The listing builds one solid part. Answer for the finished solid, in the listing's coordinates (mm). Face numbers are marked on the shaded views. A direction names the side the tool comes from. Give positions to 0.01 mm unless a question says otherwise; leave off trailing zeros. Write each loop counter-clockwise with the first axis right and the second up, starting at its lowest first coordinate (ties: lowest second). Pieces come first, ordered by that corner, then holes. Notation, with made-up numbers: (35.5, 82.5) - (70.5, 82.5) arc R20 ccw to (70.5, 103.5) - close; hole circle Ø5 at (-39, 43.5). An arc over 180 degrees is marked (long way). Answer in a Markdown table with one row per item. Add a question column.
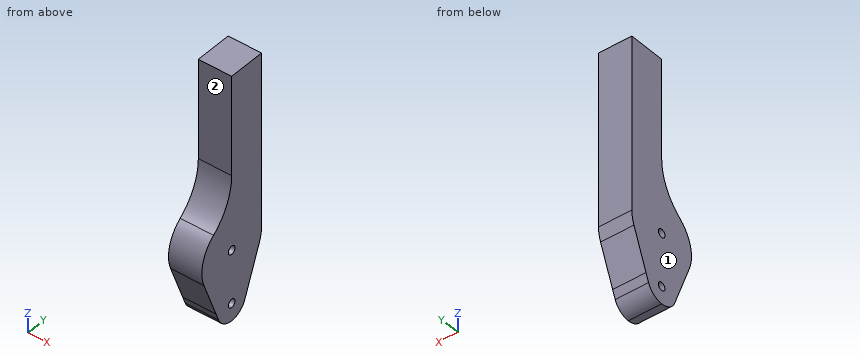
from build123d import *

# Parameters (mm, degrees)
EXTRUDE_1_DEPTH = 8.13
FILLET_1_R      = 14


with BuildPart() as part:
    # 草图1 → 凸台-拉伸1 (new body)
    with BuildSketch(Plane(origin=(0, 0, 0), x_dir=(0, 0, -1), z_dir=(1, 0, 0))):
        with BuildLine():
            Line((-30, 4.725), (4.860079961, 4.725))
            ThreePointArc((4.860079961, 4.725), (8.133942545, 7.858912138), (12.52, 9))
            Line((12.52, 9), (-30, 9))
            Line((-30, 9), (-30, 4.725))
        make_face()
        with BuildLine():
            ThreePointArc((12.52, 9), (8.133942545, 7.858912138), (4.860079961, 4.725))
            Line((4.860079961, 4.725), (20.179920039, 4.725))
            ThreePointArc((20.179920039, 4.725), (18.292906217, 6.904603813), (15.813528505, 8.375719073))
            ThreePointArc((15.813528505, 8.375719073), (14.196085968, 8.842552563), (12.52, 9))
        make_face()
        with BuildLine():
            ThreePointArc((11.52, 0), (12.52, 1), (13.52, 0))
            Line((13.52, 0), (21.25, 0))
            ThreePointArc((21.25, 0), (21.296353514, 0.625984202), (21.434402928, 1.238313549))
            ThreePointArc((21.434402928, 1.238313549), (20.988547163, 3.046917943), (20.179920039, 4.725))
            Line((20.179920039, 4.725), (4.860079961, 4.725))
            ThreePointArc((4.860079961, 4.725), (3.861498965, 2.455679097), (3.52, 0))
            Line((3.52, 0), (11.52, 0))
        make_face()
        with BuildLine():
            ThreePointArc((21.434402928, 1.238313549), (21.498575231, 0.620634213), (21.52, 0))
            Line((21.52, 0), (24.5, 0))
            ThreePointArc((24.5, 0), (25.5, 1), (26.5, 0))
            Line((26.5, 0), (29.75, 0))
            ThreePointArc((29.75, 0), (29.012294744, 2.392965865), (27.05527735, 3.955200673))
            ThreePointArc((27.05527735, 3.955200673), (23.650460817, 3.826448067), (21.434402928, 1.238313549))
        make_face()
        with BuildLine():
            Line((24.5, 0), (21.52, 0))
            ThreePointArc((21.52, 0), (21.498575231, -0.620634213), (21.434402928, -1.238313549))
            ThreePointArc((21.434402928, -1.238313549), (23.650460817, -3.826448067), (27.05527735, -3.955200673))
            ThreePointArc((27.05527735, -3.955200673), (29.012294744, -2.392965865), (29.75, 0))
            Line((29.75, 0), (26.5, 0))
            ThreePointArc((26.5, 0), (25.5, -1), (24.5, 0))
        make_face()
        with BuildLine():
            ThreePointArc((20.179920039, 4.725), (20.988547163, 3.046917943), (21.434402928, 1.238313549))
            ThreePointArc((21.434402928, 1.238313549), (23.650460817, 3.826448067), (27.05527735, 3.955200673))
            Line((27.05527735, 3.955200673), (25.097613132, 4.725))
            Line((25.097613132, 4.725), (20.179920039, 4.725))
        make_face()
        with BuildLine():
            ThreePointArc((15.813528505, 8.375719073), (18.292906217, 6.904603813), (20.179920039, 4.725))
            Line((20.179920039, 4.725), (25.097613132, 4.725))
            Line((25.097613132, 4.725), (15.813528505, 8.375719073))
        make_face()
        with BuildLine():
            Line((-30, 0), (3.52, 0))
            ThreePointArc((3.52, 0), (3.861498965, 2.455679097), (4.860079961, 4.725))
            Line((4.860079961, 4.725), (-30, 4.725))
            Line((-30, 4.725), (-30, 0))
        make_face()
        with BuildLine():
            Line((21.25, 0), (13.52, 0))
            ThreePointArc((13.52, 0), (12.52, -1), (11.52, 0))
            Line((11.52, 0), (3.52, 0))
            ThreePointArc((3.52, 0), (3.861498965, -2.455679097), (4.860079961, -4.725))
            Line((4.860079961, -4.725), (20.179920039, -4.725))
            ThreePointArc((20.179920039, -4.725), (20.988547163, -3.046917943), (21.434402928, -1.238313549))
            ThreePointArc((21.434402928, -1.238313549), (21.296353514, -0.625984202), (21.25, 0))
        make_face()
        with BuildLine():
            Line((20.179920039, -4.725), (4.860079961, -4.725))
            ThreePointArc((4.860079961, -4.725), (9.674252086, -8.538250336), (15.813528505, -8.375719073))
            ThreePointArc((15.813528505, -8.375719073), (18.292906217, -6.904603813), (20.179920039, -4.725))
        make_face()
        with BuildLine():
            ThreePointArc((27.05527735, -3.955200673), (23.650460817, -3.826448067), (21.434402928, -1.238313549))
            ThreePointArc((21.434402928, -1.238313549), (20.988547163, -3.046917943), (20.179920039, -4.725))
            Line((20.179920039, -4.725), (25.097613132, -4.725))
            Line((25.097613132, -4.725), (27.05527735, -3.955200673))
        make_face()
        with BuildLine():
            ThreePointArc((21.434402928, 1.238313549), (21.296353514, 0.625984202), (21.25, 0))
            Line((21.25, 0), (21.52, 0))
            ThreePointArc((21.52, 0), (21.498575231, 0.620634213), (21.434402928, 1.238313549))
        make_face()
        with BuildLine():
            Line((21.52, 0), (21.25, 0))
            ThreePointArc((21.25, 0), (21.296353514, -0.625984202), (21.434402928, -1.238313549))
            ThreePointArc((21.434402928, -1.238313549), (21.498575231, -0.620634213), (21.52, 0))
        make_face()
        with BuildLine():
            Line((25.097613132, -4.725), (20.179920039, -4.725))
            ThreePointArc((20.179920039, -4.725), (18.292906217, -6.904603813), (15.813528505, -8.375719073))
            Line((15.813528505, -8.375719073), (25.097613132, -4.725))
        make_face()
    extrude(amount=EXTRUDE_1_DEPTH)

    # 圆角1
    fillet_1_edges = [part.edges().sort_by_distance(p)[0] for p in [
        (4.065, 0, -3.52),
    ]]
    fillet(fillet_1_edges, radius=FILLET_1_R)


solid = part.part
1. A tool of negligible diameter and unlimited length cuts with its end or side. For the marked faces 1 and 2, from which of +Z, -Z, +X, -X, +Y, -Y can it reach the whole face along a straight path? Write none if from no direction.
2. Section B-B (z = 23) is taken. Give the vertices of the cut face in (x, y), and give its area (3 significant figures).
3. Given pin 1 Ø4 at (x, z) = (2, 15.5) entering from -Y; pin 2 Ø1 at (x, z) = (1, -6.5) entering from -Y, each flat-ended and moving along its own axis, determine where each tip first touches the part or whether it passes through.
4. Section C-C (y = 6.5) is taken. Give the vertices of the cut face in (x, z).
5. Section A-A (x = 7) is taken. State how many separate pieces and enclosed holes the cut face has, and give its area (3 significant figures).
6. Straight lines are drawn through the part: L1, parallel to Y at x = 3, z = -12.52; L2, parallel to Z at x = 7.75, y = 0.25; L3, parallel to Y at x = 0.75, z = 18.5. For each, find the intervals that lie inside material, in ascending order. Write a range as [from, to].
Geometry check:
| question | item | result |
|---|---|---|
| 1 | face 1 | +Z, -Z, -X, +Y, -Y |
| 1 | face 2 | +Z, +X, -X, -Y |
| 2 | outline | (0, 0) - (8.13, 0) - (8.13, 9) - (0, 9) - close |
| 2 | area | 73.2 mm² |
| 3 | pin 1 | y = 0 |
| 3 | pin 2 | y = -7.11 |
| 4 | outline | (0, -20.58) - (8.13, -20.58) - (8.13, 30) - (0, 30) - close |
| 5 | separate pieces | 1 |
| 5 | enclosed holes | 2 |
| 5 | area | 663 mm² |
| 6 | L1 | [-9, -1], [1, 9] |
| 6 | L2 | [-29.74, -26.47], [-24.53, -13.49], [-11.55, 30] |
| 6 | L3 | [0, 9] |
